from build123d import *

# Parameters (mm, degrees)
F1_DEPTH = 30
F2_W     = 10
F2_H     = 10
F3_DEPTH = 10
F4_T     = -2.5
F5_SIZE  = 2
F6_SIZE  = 2


with BuildPart() as f1:
    # F0 (on Front) → F1 (new body)
    with BuildSketch(Plane.XZ):
        Polygon((-60, 0), (0, 0), (0, 10), (-20, 10), (-20, 25), (-40, 25), (-40, 30), (-60, 30), align=None)
    extrude(amount=-F1_DEPTH)

    # F2 (on face) → F3 (cut)
    with BuildSketch(Plane.XZ):
        with Locations((-5, 5)):
            Rectangle(F2_W, F2_H)
    extrude(amount=-F3_DEPTH, mode=Mode.SUBTRACT)

    # F4
    f4_openings = [f1.faces().sort_by_distance(p)[0] for p in [
        (-50, 15, 30),
        (-38.75, 0, 13.125),
    ]]
    offset(amount=F4_T, openings=f4_openings, kind=Kind.INTERSECTION)

    # F5
    f5_edges = [f1.edges().sort_by_distance(p)[0] for p in [
        (-57.5, 13.75, 30),
    ]]
    chamfer(f5_edges, length=F5_SIZE)

    # F6
    f6_edges = [f1.edges().sort_by_distance(p)[0] for p in [
        (-42.5, 13.75, 22.5),
    ]]
    chamfer(f6_edges, length=F6_SIZE)


solid = f1.part
Geometry check sheet. Reference: the model listing, model coordinates, mm. A direction names the side the tool comes from. Round coordinates to 2 decimals unless told otherwise and drop trailing zeros. Order: outer loops, then holes, each group sorted by start corner. A loop starts at its lowest first (then second) coordinate and runs counter-clockwise, first axis right, second up. Notation, with made-up numbers: M 78,42 L 137,42 A10 ccw 137,61 Z; hole C 54.5,-39 d3. An arc over 180 degrees is marked long. Write each question's results on one line, items separated by ' | '. Start each with the question number.
1. Cross-section at A-A on z = 14. Record the boundary of the cut face in (x, y), plus the area to 4 significant figures.
2. Cross-section at B-B on y = 2.5. Record the boundary of the cut face in (x, z).
3. Material ranges on L1, parallel to X at y = 10.25, z = 9; L2, parallel to X at y = 9.25, z = 8; L3, parallel to Z at x = -35.5, y = 10.5, recorded low to high. Write a range as from..to.
4. Cross-section at C-C on x = -18.5. Record the boundary of the cut face in (y, z), plus the area to 4 significant figures.
5. Go/stop test with flat-tipped pins: P1, Ø16, axis at x = -29, y = 11.5, coming from the +Z side; P2, Ø10, axis at x = -16.5, y = 7, coming from the -Z side; P3, Ø12, axis at y = 11, z = 17.5, coming from the +X side; P4, Ø8, axis at x = -3, z = 6.5, coming from the -Y side. Record where each tip stops, or that it passes through.
6. Set-up check for faces 1 (the face through (-40, 15, 27)), 2 (the face through (-42.5, 14, 27)), 3 (the face through (-8, 12.5, 5)): record each of +Z, -Z, +X, -X, +Y, -Y from which the full face is reachable in a straight line by a thin tool's end or side.
7. Cross-section at D-D on z = 6.75. Record the boundary of the cut face in (x, y).
8. Draft check along Y on faces 4 (the face through (-35, 0, 2)), 5 (the face through (-12.5, 6, 5)), 6 (the face through (-2.5, 20, 5)). Enter one of: pulls with the +Y half, pulls with the -Y half, needs draft (parallel to the pull), parting line crosses it, or undercut.
Resolved:
1) outline: M -60,0 L -57.5,0 L -57.5,27.5 L -22.5,27.5 L -22.5,0 L -20,0 L -20,30 L -60,30 Z | area: 237.5 mm2
2) outline: M -60,0 L -10,0 L -10,10 L -20,10 L -20,25 L -40,25 L -40,30 L -42.5,30 L -42.5,24.5 L -40.5,22.5 L -22.5,22.5 L -22.5,7.5 L -12.5,7.5 L -12.5,2.5 L -57.5,2.5 L -57.5,28 L -59.5,30 L -60,30 Z
3) L1: -60..-57.5, -22.5..0 | L2: -60..-57.5, -22.5..-10 | L3: 0..2.5, 22.5..25
4) outline: M 0,0 L 30,0 L 30,10 L 0,10 L 0,7.5 L 27.5,7.5 L 27.5,2.5 L 0,2.5 Z | area: 162.5 mm2
5) P1: z = 25 | P2: z = 0 | P3: x = -20 | P4: y = 10
6) face 1: +Z, +X, +Y, -Y | face 2: +Z, -Y | face 3: none
7) outline: M -60,0 L -57.5,0 L -57.5,27.5 L -2.5,27.5 L -2.5,12.5 L -12.5,12.5 L -12.5,0 L -10,0 L -10,10 L 0,10 L 0,30 L -60,30 Z
8) face 4: pulls with the -Y half | face 5: needs draft | face 6: undercut
